```python
from build123d import *

# Parameters (mm, degrees)
SKETCH1_W           = 32
SKETCH1_H           = 11.5
BOSS_EXTRUDE1_DEPTH = 2
SKETCH2_R           = 1.5
CUT_EXTRUDE1_DEPTH  = 35.062442661
FILLET1_R           = 4
SKETCH3_W           = 2
SKETCH3_H           = 3
BOSS_EXTRUDE2_DEPTH = 1.5


with BuildPart() as part:
    # Sketch1 → Boss-Extrude1 (new body)
    with BuildSketch(Plane(origin=(0, 0, 0), x_dir=(1, 0, 0), z_dir=(0, 1, 0))):
        with Locations((16, -5.75)):
            Rectangle(SKETCH1_W, SKETCH1_H)
    extrude(amount=BOSS_EXTRUDE1_DEPTH)

    # Sketch2 → Cut-Extrude1 (cut, through all)
    with BuildSketch(Plane(origin=(0, 2, 0), x_dir=(1, 0, 0), z_dir=(0, 1, 0))):
        with Locations(Location((3, -5.75, 0), (0, 0, 270))):
            Circle(SKETCH2_R)
        with Locations(Location((29, -5.75, 0), (0, 0, 270))):
            Circle(SKETCH2_R)
    extrude(amount=-CUT_EXTRUDE1_DEPTH, mode=Mode.SUBTRACT)

    # Fillet1
    fillet1_edges = [part.edges().sort_by_distance(p)[0] for p in [
        (0, 1, 0),
        (32, 1, 0),
        (32, 1, 11.5),
        (0, 1, 11.5),
    ]]
    fillet(fillet1_edges, radius=FILLET1_R)

    # Sketch3 → Boss-Extrude2 (add)
    with BuildSketch(Plane(origin=(0, 2, 0), x_dir=(1, 0, 0), z_dir=(0, 1, 0))):
        with Locations((12, -5.75)):
            Rectangle(SKETCH3_W, SKETCH3_H)
        with Locations((20, -5.75)):
            Rectangle(SKETCH3_W, SKETCH3_H)
    extrude(amount=BOSS_EXTRUDE2_DEPTH)


solid = part.part
```
Geometry check sheet. Reference: the model listing, model coordinates, mm. A direction names the side the tool comes from. Give positions to 0.01 mm unless a question says otherwise; leave off trailing zeros. Write each loop counter-clockwise with the first axis right and the second up, starting at its lowest first coordinate (ties: lowest second). Pieces come first, ordered by that corner, then holes. Notation, with made-up numbers: (-39, 13) -> (11, 13) arc R20 ccw to (11, 37) -> close; hole circle Ø5 at (57, 8.5). An arc over 180 degrees is marked (long way). One line per question, with ' | ' between items.
Item 1: Sectioned sample at A-A, the plane z = 5.75. Record the boundary of the cut face in (x, y).
Determined:
outline: (0, 0) -> (1.5, 0) -> (1.5, 2) -> (0, 2) -> close; (4.5, 0) -> (27.5, 0) -> (27.5, 2) -> (21, 2) -> (21, 3.5) -> (19, 3.5) -> (19, 2) -> (13, 2) -> (13, 3.5) -> (11, 3.5) -> (11, 2) -> (4.5, 2) -> close; (30.5, 0) -> (32, 0) -> (32, 2) -> (30.5, 2) -> close
Item 2: Sectioned sample at B-B, the plane y = 1.7. Record the boundary of the cut face in (x, z).
Determined:
outline: (0, 4) arc R4 ccw to (4, 0) -> (28, 0) arc R4 ccw to (32, 4) -> (32, 7.5) arc R4 ccw to (28, 11.5) -> (4, 11.5) arc R4 ccw to (0, 7.5) -> close; hole circle Ø3 at (3, 5.75); hole circle Ø3 at (29, 5.75)
Item 3: Sectioned sample at D-D, the plane x = 9.5. Record the boundary of the cut face in (y, z), plus the area to 3 significant figures.
Determined:
outline: (0, 0) -> (2, 0) -> (2, 11.5) -> (0, 11.5) -> close | area: 23.0 mm^2
Item 4: Depth check by flat-ended pin: pin 1 (5 mm diameter, centred on x = 18, z = 7.5, fed in from -Y); pin 2 (0.8 mm diameter, centred on x = 20.5, y = 3, fed in from -Z); pin 3 (2 mm diameter, centred on y = 0.5, z = 10.5, fed in from +X); pin 4 (1.6 mm diameter, centred on x = 11.5, y = 3, fed in from +Z). Enter the tip coordinate at first touch or a pass-through.
Determined:
pin 1: y = 0 | pin 2: z = 4.25 | pin 3: x = 31.46 | pin 4: z = 7.25
Item 5: Scan lines: line 1 along X through (y, z) = (1.8, 5.75); line 2 along X through (y, z) = (2.65, 6); line 3 along Y through (x, z) = (27.5, 3.5). Record each from-to range of solid material in increasing order.
Determined:
line 1: 0 to 1.5, 4.5 to 27.5, 30.5 to 32 | line 2: 11 to 13, 19 to 21 | line 3: 0 to 2
Item 6: Sectioned sample at C-C, the plane x = 29. Record the boundary of the cut face in (y, z).
Determined:
outline: (0, 0.13) -> (2, 0.13) -> (2, 4.25) -> (0, 4.25) -> close; (0, 7.25) -> (2, 7.25) -> (2, 11.37) -> (0, 11.37) -> close
Item 7: Draft check along Z on faces 4 (the cylindrical face through (1.141, 1.014, 1.203)), 5 (the flat face through (12, 3.5, 6)), 6 (the cylindrical face through (1.141, 1.014, 10.297)), 7 (the cylindrical face through (30.487, 1.014, 5.555)). Enter one of: released by +Z, released by -Z, zero draft, split by the parting line, or undercut.
Determined:
face 4: released by -Z | face 5: zero draft | face 6: released by +Z | face 7: undercut
Item 8: Access from +Z, -Z, +X, -X, +Y, -Y to the whole of each face (thin tool, end or side, straight path). Record for faces 1 (the flat face through (19, 3, 6)), 2 (the flat face through (12, 3, 4.25)), 3 (the flat face through (21, 3, 6)).
Determined:
face 1: +Z, -Z, +Y | face 2: -Z, +X, -X, +Y | face 3: +Z, -Z, +X, +Y
